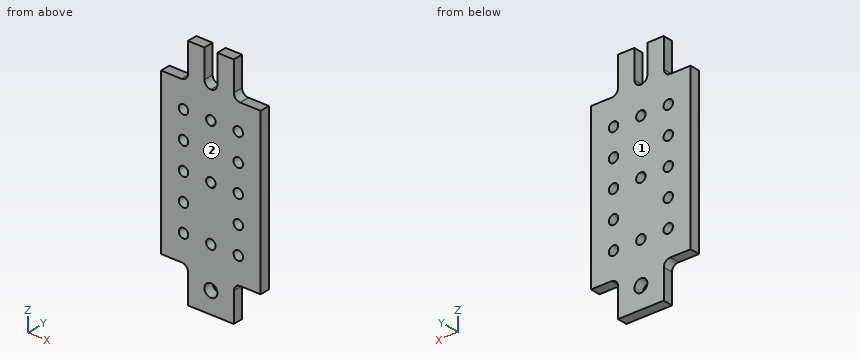
from build123d import *

# Parameters (mm, degrees)
F1_DEPTH = 10
F3_D     = 9.5
F7_D     = 13
F8_R     = 6.49999
F9_R     = 6.5


# Not quite as in the source:
# - a fillet or chamfer is up to 0.001 mm smaller than in the source, because OpenCascade refuses the exact size


with BuildPart() as f1:
    # F0 (on Front) → F1 (new body)
    with BuildSketch(Plane.XZ):
        Polygon((-23, 0), (0, 0), (0, 200), (-6.5, 200), (-6.5, 235), (-23, 235), (-23, 199), (-50, 199), (-50, 36), (-23, 36), align=None)
    extrude(amount=F1_DEPTH)

    # F3 (through all)
    with Locations(Plane.XZ.offset(10)):
        with Locations((-27.5, 172.5), (-27.5, 145), (-27.5, 117.5), (-27.5, 90), (-27.5, 62.5), (0, 62.5), (0, 117.5), (0, 172.5)):
            Hole(F3_D / 2)

    # F4: F1 across face


with BuildPart() as f1_1:
    add(f1.part)
    add(f1.part.mirror(Plane(origin=(0, -5, 90), x_dir=(0, 1, 0), z_dir=(1, 0, 0))))

    # F7 (through all)
    with Locations(Plane.XZ.offset(10)):
        with Locations((0, 21.5)):
            Hole(F7_D / 2)

    # F8 (radius 6.5 in the source; OpenCascade refuses exactly that, so slightly less here)
    f8_edges = [f1_1.edges().sort_by_distance(p)[0] for p in [
        (-6.5, -5, 200),
        (6.5, -5, 200),
    ]]
    fillet(f8_edges, radius=F8_R)

    # F9
    f9_edges = [f1_1.edges().sort_by_distance(p)[0] for p in [
        (23, -5, 199),
        (-23, -5, 199),
        (23, -5, 36),
        (-23, -5, 36),
    ]]
    fillet(f9_edges, radius=F9_R)


solid = f1_1.part
For this review, take the finished solid that the model builds, in its own axes (mm). Face numbers are marked on the shaded views. Round coordinates to 2 decimals unless told otherwise and drop trailing zeros. Loops run counter-clockwise (first coordinate to the right, second up) from the corner with the lowest first, then second, coordinate; pieces in that order, holes last. Notation, with made-up numbers: (60.5, 43.25) - (113.5, 43.25) arc R10 cw to (113.5, 61.25) - close; hole circle Ø5 at (0, 53). An arc over 180 degrees is marked (long way). One line per item, written item: value. Start each with the question number.
Item 1: For L1, parallel to Z at x = -27.5, y = -2.5; L2, parallel to Z at x = -3, y = -2; L3, parallel to X at y = -5.5, z = 144, list the stretches that pass through material, from the lowest coordinate up.
Item 2: The part is to be moulded in two halves that separate along Y. For the marked faces 1 and 2, say which applies: +Y half, -Y half, draft (parallel to the pull), parting line (faces both ways), or undercut.
Item 3: Take a section at A-A (z = 145). Give the boundary of the cut face in (x, y).
Item 4: Clearance check with flat-ended pins moving along their axes: pin 1 Ø1.5 at (x, y) = (1.5, -2) entering from +Z; pin 2 Ø3 at (y, z) = (-3.5, 214.5) entering from -X; pin 3 Ø6 at (x, y) = (37.5, -6.5) entering from -Z. State where each tip first meets the part, or that it passes through.
Item 5: Take a section at B-B (z = 209). Give the boundary of the cut face in (x, y).
Item 6: Take a section at C-C (z = 117.5). Give the boundary of the cut face in (x, y), plus the area to 3 significant figures.
Item 7: Take a section at D-D (x = 41.5). Give the boundary of the cut face in (y, z).
Answer below:
1. L1: z = 35.68 to 57.75, 67.25 to 85.25, 94.75 to 112.75, 122.25 to 140.25, 149.75 to 167.75, 177.25 to 199.32
1. L2: z = 0 to 15.73, 27.27 to 58.82, 66.18 to 113.82, 121.18 to 168.82, 176.18 to 200.73
1. L3: x = -50 to -32.14, -22.86 to 22.86, 32.14 to 50
2. face 1: +Y half
2. face 2: -Y half
3. outline: (-50, -10) - (-32.25, -10) - (-32.25, 0) - (-50, 0) - close; (-22.75, -10) - (22.75, -10) - (22.75, 0) - (-22.75, 0) - close; (32.25, -10) - (50, -10) - (50, 0) - (32.25, 0) - close
4. pin 1: stops at z = 200.4
4. pin 2: stops at x = -23
4. pin 3: stops at z = 36
5. outline: (-23, -10) - (-6.5, -10) - (-6.5, 0) - (-23, 0) - close; (6.5, -10) - (23, -10) - (23, 0) - (6.5, 0) - close
6. outline: (-50, -10) - (-32.25, -10) - (-32.25, 0) - (-50, 0) - close; (-22.75, -10) - (-4.75, -10) - (-4.75, 0) - (-22.75, 0) - close; (4.75, -10) - (22.75, -10) - (22.75, 0) - (4.75, 0) - close; (32.25, -10) - (50, -10) - (50, 0) - (32.25, 0) - close
6. area: 715 mm2
7. outline: (-10, 36) - (0, 36) - (0, 199) - (-10, 199) - close
